For this review, take the finished solid that the model builds, in its own axes (mm). A direction names the side the tool comes from. Give positions to 0.01 mm unless a question says otherwise; leave off trailing zeros. Loops run counter-clockwise (first coordinate to the right, second up) from the corner with the lowest first, then second, coordinate; pieces in that order, holes last. Notation, with made-up numbers: (-20, 34) - (5, 34) arc R18 cw to (5, 64) - close; hole circle Ø6 at (12.25, 37). An arc over 180 degrees is marked (long way). Put each result on its own line as item: value.
from build123d import *

# Parameters (mm, degrees)
F0_W     = 25.4
F0_H     = 25.4
F1_DEPTH = 25.4
F3_DEPTH = 412.75
F5_DEPTH = 598.932


with BuildPart() as f1:
    # F0 (on Front) → F1 (new body)
    with BuildSketch(Plane.XZ):
        Polygon((-203.2, -57.15), (203.2, -57.15), (203.2, 31.75), (177.8, 31.75), (152.4, 31.75), (127, 31.75), (101.6, 31.75), (76.2, 31.75), (50.8, 31.75), (25.4, 31.75), (0, 31.75), (-25.4, 31.75), (-50.8, 31.75), (-76.2, 31.75), (-101.6, 31.75), (-127, 31.75), (-152.4, 31.75), (-177.8, 31.75), (-203.2, 31.75), align=None)
        with Locations((190.5, 44.45)):
            Rectangle(F0_W, F0_H)
        with Locations((139.7, 44.45)):
            Rectangle(F0_W, F0_H)
        with Locations((88.9, 44.45)):
            Rectangle(F0_W, F0_H)
        with Locations((38.1, 44.45)):
            Rectangle(F0_W, F0_H)
        with Locations((-12.7, 44.45)):
            Rectangle(F0_W, F0_H)
        with Locations((-63.5, 44.45)):
            Rectangle(F0_W, F0_H)
        with Locations((-114.3, 44.45)):
            Rectangle(F0_W, F0_H)
        with Locations((-165.1, 44.45)):
            Rectangle(F0_W, F0_H)
    extrude(amount=F1_DEPTH)

    # F2 (on face) → F3 (cut)
    with BuildSketch(Plane.YZ.offset(203.2)):
        with BuildLine():
            ThreePointArc((-4.617769491, 52.532230509), (-8.5240978333, 54.3652091128), (-12.7, 53.278446593))
            Line((-12.7, 53.278446593), (-12.7, 50.8))
            ThreePointArc((-12.7, 50.8), (-10.2699602045, 50.3166350314), (-8.2098719395, 48.9401280605))
            Line((-8.2098719395, 48.9401280605), (-4.617769491, 52.532230509))
        make_face()
        with BuildLine():
            Line((-12.7, 50.8), (-12.7, 53.278446593))
            ThreePointArc((-12.7, 53.278446593), (-14.0784278664, 51.9938524898), (-15.0192191193, 50.3613215677))
            ThreePointArc((-15.0192191193, 50.3613215677), (-13.8801711836, 50.6893666327), (-12.7, 50.8))
        make_face()
        with BuildLine():
            ThreePointArc((-8.2098719395, 48.9401280605), (-10.2699602045, 50.3166350314), (-12.7, 50.8))
            Line((-12.7, 50.8), (-12.7, 44.45))
            Line((-12.7, 44.45), (-8.2098719395, 48.9401280605))
        make_face()
        with BuildLine():
            Line((-12.7, 44.45), (-12.7, 50.8))
            ThreePointArc((-12.7, 50.8), (-13.8801711836, 50.6893666327), (-15.0192191193, 50.3613215677))
            ThreePointArc((-15.0192191193, 50.3613215677), (-15.3239526387, 46.744736211), (-13.5980256121, 43.5519743879))
            Line((-13.5980256121, 43.5519743879), (-12.7, 44.45))
        make_face()
        with BuildLine():
            ThreePointArc((-13.5980256121, 43.5519743879), (-15.3239526387, 46.744736211), (-15.0192191193, 50.3613215677))
            ThreePointArc((-15.0192191193, 50.3613215677), (-18.9160550871, 45.7473662374), (-17.1901280605, 39.9598719395))
            Line((-17.1901280605, 39.9598719395), (-13.5980256121, 43.5519743879))
        make_face()
        with BuildLine():
            Line((-8.2098719395, 48.9401280605), (-12.7, 44.45))
            Line((-12.7, 44.45), (-13.5980256121, 43.5519743879))
            Line((-13.5980256121, 43.5519743879), (-9.1986165609, 39.1525653367))
            ThreePointArc((-9.1986165609, 39.1525653367), (-7.1073134882, 41.4426161567), (-6.35, 44.45))
            ThreePointArc((-6.35, 44.45), (-6.8333649686, 46.8800397955), (-8.2098719395, 48.9401280605))
        make_face()
        with BuildLine():
            Line((-13.5980256121, 43.5519743879), (-17.1901280605, 39.9598719395))
            ThreePointArc((-17.1901280605, 39.9598719395), (-13.3382319087, 38.1321554284), (-9.1986165609, 39.1525653367))
            Line((-9.1986165609, 39.1525653367), (-13.5980256121, 43.5519743879))
        make_face()
        with BuildLine():
            Line((0, 40.7302561211), (-8.2098719395, 48.9401280605))
            ThreePointArc((-8.2098719395, 48.9401280605), (-6.8333649686, 46.8800397955), (-6.35, 44.45))
            ThreePointArc((-6.35, 44.45), (-7.1073134882, 41.4426161567), (-9.1986165609, 39.1525653367))
            Line((-9.1986165609, 39.1525653367), (0, 29.9539487758))
            Line((0, 29.9539487758), (0, 40.7302561211))
        make_face()
        Polygon((0, 47.9144610179), (-4.617769491, 52.532230509), (-8.2098719395, 48.9401280605), (0, 40.7302561211), align=None)
    extrude(amount=-F3_DEPTH, mode=Mode.SUBTRACT)

    # F4 (on face) → F5 (cut)
    with BuildSketch(Plane.YZ.offset(203.2)):
        with BuildLine():
            ThreePointArc((-12.7, -55.245), (-8.6588847455, -53.5711152545), (-6.985, -49.53))
            ThreePointArc((-6.985, -49.53), (-16.7411152545, -45.4888847455), (-12.7, -55.245))
        make_face()
    extrude(amount=-F5_DEPTH, mode=Mode.SUBTRACT)


solid = f1.part
1) Take a section at B-B on x = 12. State the section outline as (y, z) points (3 decimals), and give its area (3 significant figures).
Geometry check:
outline: (-25.4, -57.15) - (0, -57.15) - (0, 29.954) - (-1.796, 31.75) - (-25.4, 31.75) - close; hole circle Ø11.43 at (-12.7, -49.53)
area: 2,150 mm²
2) Wall thickness on line 1 (Z direction, x = -22.5, y = -12.7) (3 decimals); line 2 (Z direction, x = 52, y = -12.7) (3 decimals); line 3 (Y direction, x = 88, z = -50.5): over which ranges is each line inside the solid? List them lowest first.
Geometry check:
line 1: z = -57.15 to -55.245, -43.815 to 38.1, 53.278 to 57.15
line 2: z = -57.15 to -55.245, -43.815 to 31.75
line 3: y = -25.4 to -18.33, -7.07 to 0
3) For faces 4 (the face through (48, -3.642, 33.596)), 5 (the face through (38, 0, 53)), 6 (the face through (101.6, -21, 44)), list the 3-axis set-ups (+Z, -Z, +X, -X, +Y, -Y) from which the entire face can be reached by the end or side of a thin tool; tool diameter is ignored.
Geometry check:
face 4: +X, -X, +Y
face 5: +Z, -Z, +X, -X, +Y
face 6: +Z, +Y, -Y
4) Draft analysis for pull direction X (two halves, no side actions). For faces 1 (the face through (89, 0, 53)), 2 (the face through (203.2, -13, -1)), 3 (the face through (152.4, -21, 44)), state which applies: pulls with the +X half, pulls with the -X half, needs draft (parallel to the pull), parting line crosses it, or undercut.
Geometry check:
face 1: needs draft
face 2: pulls with the +X half
face 3: undercut
5) Insertion check: pin 1 Ø1 at (x, z) = (-111, 34.5) entering from +Y; pin 2 Ø12 at (x, y) = (62, -13) entering from +Z; pin 3 Ø12.5 at (y, z) = (-11, 41.5) entering from -X. Each pin has a flat end and moves straight along its axis. Give the tip position at first contact, or say it passes through.
Geometry check:
pin 1: stops at y = -4.05
pin 2: stops at z = 31.75
pin 3: stops at x = -177.8
6) Take a section at A-A on x = 94.5. State the section outline as (y, z) points (3 decimals), and give its area (3 significant figures).
Geometry check:
outline: (-25.4, -57.15) - (0, -57.15) - (0, 29.954) - (-9.199, 39.153) arc R6.35 cw (long way) to (-15.019, 50.361) arc R6.35 cw to (-4.618, 52.532) - (0, 47.914) - (0, 57.15) - (-25.4, 57.15) - close; hole circle Ø11.43 at (-12.7, -49.53)
area: 2,520 mm²
